Design review of the part built by this model. Coordinates are the model's own, in mm. Give positions to 0.01 mm unless a question says otherwise; leave off trailing zeros. Loops run counter-clockwise (first coordinate to the right, second up) from the corner with the lowest first, then second, coordinate; pieces in that order, holes last. Notation, with made-up numbers: (-31.5, -4) -> (7.5, -4) arc R19 ccw to (7.5, 9) -> close; hole circle Ø2 at (-5, 61.25). An arc over 180 degrees is marked (long way). Answer in a Markdown table with one row per item. Add a question column.
(1) Consider section A-A on z = 0. Write out the cut boundary in (x, y).
(2) Consider section B-B on x = -127.5. Write out the cut boundary in (y, z).
(3) For pin 1 (8 mm diameter, centred on x = -126.5, y = 1.5, fed in from -Z); pin 2 (1.5 mm diameter, centred on x = -61.5, y = -4, fed in from -Z); pin 3 (10 mm diameter, centred on x = -78, y = 5.5, fed in from +Z), all flat-tipped, find the tip position at first contact; note any pin that passes through.
(4) For line 1 (X direction, y = -3.25, z = 0); line 2 (Y direction, x = -32, z = -34); line 3 (X direction, y = 7, z = -120.5), list the stretches that pass through material, from the lowest coordinate up.
(5) Consider section C-C on z = -62.5. Write out the cut boundary in (x, y).
(6) Consider section D-D on x = -56.5. Write out the cut boundary in (y, z).
Autodesk Inventor part; units mm, degrees
ref_plane "YZ Plane" through (0, 0, 0) normal (1, 0, 0) x (0, 1, 0)
ref_plane "XZ Plane" through (0, 0, 0) normal (0, 1, 0) x (-1, 0, 0)
ref_plane "XY Plane" through (0, 0, 0) normal (0, 0, 1) x (1, 0, 0)
sketch "Sketch1" plane through (0, 0, 0) normal (0, 1, 0) x (-1, 0, 0)
  circle A0 centre (0, 0) radius 135
  circle A1 centre (0, 0) radius 110
  dimension "d0" = 270
  dimension "d1" = 220
extrude "Extrusion1" add sketch "Sketch1" along normal mid plane 20
sketch "Sketch2" plane through (0, 10, 0) normal (0, 1, 0) x (1, 0, 0)
  circle A0 centre (0, 0) radius 37.5
  circle A1 centre (0, 0) radius 135
  dimension "d4" = 75
  dimension "d20" = 270
extrude "Extrusion2" add sketch "Sketch2" against normal blind 1
sketch "Sketch3" plane through (0, 10, 0) normal (0, 1, 0) x (1, 0, 0)
  circle A0 centre (0, 0) radius 127.5
  circle A1 centre (127.5, 0) radius 2.5
  circle A2 centre (103.1497, 74.9426) radius 2.5
  circle A3 centre (39.3997, 121.2597) radius 2.5
  circle A4 centre (-39.3997, 121.2597) radius 2.5
  circle A5 centre (-103.1497, 74.9426) radius 2.5
  circle A6 centre (-127.5, 0) radius 2.5
  circle A7 centre (-103.1497, -74.9426) radius 2.5
  circle A8 centre (-39.3997, -121.2597) radius 2.5
  circle A9 centre (39.3997, -121.2597) radius 2.5
  circle A10 centre (103.1497, -74.9426) radius 2.5
  dimension "d7" = 255
  dimension "d8" = 5
  dimension "d11" = 360
hole "Hole1" at (127.5, 10, 0) at (103.1497, 10, 74.9426) at (39.3997, 10, 121.2597) at (-39.3997, 10, 121.2597) at (-103.1497, 10, 74.9426) at (-127.5, 10, 0) at (-103.1497, 10, -74.9426) at (-39.3997, 10, -121.2597) at (39.3997, 10, -121.2597) at (103.1497, 10, -74.9426) direction (0, -1, 0) diameter 5 end through all
sketch "Sketch4" plane through (0, -10, 0) normal (0, -1, 0) x (1, 0, 0)
  circle A0 centre (0, 0) radius 135
  line L0 (0, 0) -> (132.949, -23.4425)
  line L1 (0, 0) -> (135, 0) construction
  line L2 (0, 0) -> (-23.4425, -132.949)
  circle A1 centre (0, 0) radius 135
  line L3 (0, 0) -> (135, 0) construction
  line L4 (0, 0) -> (-132.949, 23.4425)
  dimension "d21" = 135
  dimension "d22" = 10
  dimension "d23" = 100
extrude "Extrusion3" cut sketch "Sketch4" against normal through all contours A0 L0 L4 | A0 L2 L0
sketch "Sketch5" plane through (-23.4425, -10, -132.949) normal (0.9848, 0, -0.1736) x (-0.1736, 0, -0.9848)
  line L0 (0, 0) -> (-25, 0)
  line L1 (-2.5, 0) -> (15, 0)
  line L2 (20, 5) -> (20, 15)
  line L3 (15, 20) -> (-2.5, 20)
  line L4 (-2.5, 20) -> (-2.5, 0)
  line L5 (0, 20) -> (0, 0)
  arc A0 (20, 15) -> (15, 20) centre (15, 15) ccw
  arc A1 (15, 0) -> (20, 5) centre (15, 5) ccw
  point P0 (-135, 10)
  point P1 (20, 20)
  point P2 (20, 0)
  point P3 (0, 0)
  dimension "d26" = 22.5
  dimension "d27" = 20
  dimension "d28" = 20
  dimension "d29" = 5
extrude "Extrusion4" add sketch "Sketch5" against normal blind 10
fillet "Fillet1" radius 2.5 1 edges at (-33.2262, 0, -130.8473)
sketch "Sketch6" plane through (-132.949, -10, 23.4425) normal (0.1736, 0, 0.9848) x (0.9848, 0, -0.1736)
  line L0 (25, 0) -> (0, 0)
  line L1 (2.5, 0) -> (-15, 0)
  line L2 (-20, 5) -> (-20, 15)
  line L3 (-15, 20) -> (2.5, 20)
  line L4 (2.5, 20) -> (2.5, 0)
  line L5 (0, 0) -> (0, 20)
  arc A0 (-15, 20) -> (-20, 15) centre (-15, 15) ccw
  arc A1 (-20, 5) -> (-15, 0) centre (-15, 5) ccw
  point P0 (135, 10)
  point P1 (-20, 20)
  point P2 (-20, 0)
  point P3 (0, 0)
  dimension "d33" = 22.5
  dimension "d34" = 20
  dimension "d35" = 20
  dimension "d36" = 5
extrude "Extrusion5" add sketch "Sketch6" against normal blind 10
fillet "Fillet2" radius 2.5 1 edges at (-134.3203, 0, 13.53)
sketch "Sketch7" plane through (-33.2906, -10, -131.2126) normal (-0.9848, 0, 0.1736) x (0.1736, 0, 0.9848)
  line L0 (-1.9306, 20) -> (-15, 20)
  line L1 (-20, 15) -> (-20, 5)
  point P0 (135, 10)
  point P1 (-10, 10)
  dimension "d40" = 10
  dimension "d41" = 10
hole "Hole2" at (-35.0271, 0, -141.0606) direction (0.9848, 0, -0.1736) diameter 8.2 end through all counterbore diameter 13.2 counterbore depth 6
sketch "Sketch8" plane through (-134.6855, -10, 13.5944) normal (-0.1736, 0, -0.9848) x (-0.9848, 0, 0.1736)
  line L0 (12.7338, 3.4) -> (7.2662, 3.4)
  line L1 (7.2662, 3.4) -> (3.4, 7.2662)
  line L2 (3.4, 7.2662) -> (3.4, 12.7338)
  line L3 (3.4, 12.7338) -> (7.2662, 16.6)
  line L4 (7.2662, 16.6) -> (12.7338, 16.6)
  line L5 (12.7338, 16.6) -> (16.6, 12.7338)
  line L6 (16.6, 12.7338) -> (16.6, 7.2662)
  line L7 (16.6, 7.2662) -> (12.7338, 3.4)
  line L8 (1.9306, 0) -> (15, 0)
  line L9 (20, 5) -> (20, 15)
  point P0 (-135, 10)
  point P1 (10, 10)
  dimension "d49" = 10
  dimension "d50" = 10
  dimension "d51" = 13.2
extrude "Extrusion6" cut sketch "Sketch8" against normal blind 6
sketch "Sketch9" plane through (-133.6436, -10, 19.5033) normal (-0.1736, 0, -0.9848) x (-0.9848, 0, 0.1736)
  line L0 (1.9306, 0) -> (15, 0)
  line L1 (20, 5) -> (20, 15)
  point P0 (-135, 10)
  point P1 (10, 10)
  dimension "d54" = 10
  dimension "d55" = 10
hole "Hole3" at (-143.4917, 0, 21.2398) direction (0.1736, 0, 0.9848) diameter 8.2 end through all
properties part number "Cylinder Spacer 25mm_Q1+3"
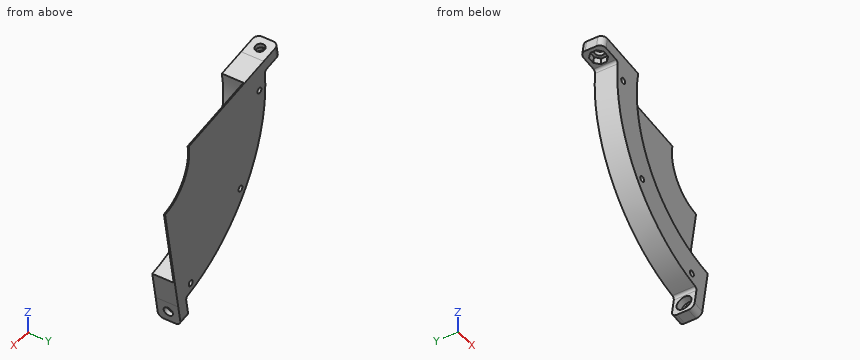
Values follow:
| question | item | result |
|---|---|---|
| 1 | outline | (-135, -10) -> (-130, -10) -> (-130, 10) -> (-135, 10) -> close; (-125, -10) -> (-110, -10) -> (-110, 9) -> (-37.5, 9) -> (-37.5, 10) -> (-125, 10) -> close |
| 2 | outline | (-10, -44.37) -> (10, -44.37) -> (10, -2.5) -> (-10, -2.5) -> close; (-10, 2.5) -> (10, 2.5) -> (10, 22.48) -> (-10, 22.48) -> close |
| 3 | pin 1 | z = -56.73 |
| 3 | pin 2 | z = -120.56 |
| 3 | pin 3 | z = 14.38 |
| 4 | line 1 | -135 to -130, -125 to -110 |
| 4 | line 2 | 9 to 10 |
| 4 | line 3 | -60.87 to -41.78, -37.02 to -21.25 |
| 5 | outline | (-119.66, -10) -> (-90.52, -10) -> (-90.52, 9) -> (-11.02, 9) -> (-11.02, 10) -> (-119.66, 10) -> close |
| 6 | outline | (-10, -122.61) -> (10, -122.61) -> (10, 9.96) -> (9, 9.96) -> (9, -94.38) -> (-10, -94.38) -> close |
